Could you check a few things on this model? Use its own coordinates, in mm. A direction names the side the tool comes from. Coordinates: 2 decimals unless noted, no trailing zeros. Write each loop counter-clockwise with the first axis right and the second up, starting at its lowest first coordinate (ties: lowest second). Pieces come first, ordered by that corner, then holes.
Item 1: Which directions (+Z, -Z, +X, -X, +Y, -Y) give clear straight access to the entire face, cutting with the end or side of a thin tool? Please do faces 5 (the flat face through (4, 24, 34)), 6 (the flat face through (4, 29, -32)), 7 (the flat face through (4, 31.5, 0)).
Item 2: If I drill on probe 1 along Y at (x, z) = (4, 34.25); probe 2 along Z at (x, y) = (2, 30.5); probe 3 along Z at (x, y) = (5.75, 19.5), over which ranges is the centre line in solid material (lowest first)?
Item 3: I want a section at D-D on x = 4. State how many separate pieces and enclosed holes the cut face has, then the cut area to 3 significant figures.
Item 4: I want a section at C-C on y = 16. Please give me the cut outline in (x, z).
Item 5: I want a section at B-B on y = 30.75. Please give me the cut outline in (x, z), then the cut area to 3 significant figures.
Item 6: I want a section at A-A on z = -24. Please give me the cut outline in (x, y).
Item 7: Thinking about a two-plate mould opening in X: for faces 1 (the cylindrical face through (4, 10, 35)), 2 (the flat face through (8, 33, -2)), 3 (the flat face through (0, 33, -2)), 4 (the flat face through (4, 21, 31)), which applies, +X half, -X half, draft (parallel to the pull), parting line (faces both ways), or undercut?
Item 8: For P1, Ø2, axis at x = 6, z = -30.5, coming from the -Y side; P2, Ø3, axis at x = 3, y = 27.5, coming from the +Z side; P3, Ø8, axis at y = 17.5, z = -26.5, coming from the -X side; P4, Ø4, axis at x = 4, z = 24, coming from the -Y side, each with a flat end and sliding along its axis, tell me the tip position at first contact or that it passes through.
from build123d import *

# Parameters (mm, degrees)
F1_DEPTH = 8
F2_W     = 6.02
F2_H     = 5
F3_DEPTH = 72
F4_R     = 1.5
F5_DEPTH = 25
F6_R     = 2
F7_DEPTH = 72
F8_SIZE  = 1


with BuildPart() as f1:
    # F0 (on Right) → F1 (new body)
    with BuildSketch(Plane.YZ):
        Polygon((24, 36), (4, 36), (4, 33), (21, 33), (21, 29), (31.5, 29), (31.5, -29), (21, -29), (21, -33), (4, -33), (4, -36), (24, -36), (24, -32), (34, -32), (34, -15.6872682273), (34, 32), (24, 32), align=None)
    extrude(amount=F1_DEPTH)

    # F2 (on face) → F3 (cut)
    with BuildSketch(Plane.XY.offset(36)):
        with Locations((3.01, 1.5)):
            Rectangle(F2_W, F2_H)
    extrude(amount=-F3_DEPTH, mode=Mode.SUBTRACT)

    # F4 (on face) → F5 (cut)
    with BuildSketch(Plane(origin=(0, 34, 0), x_dir=(-1, 0, 0), z_dir=(0, 1, 0))):
        with Locations((-4, 24)):
            Circle(F4_R)
        with Locations((-4, -24)):
            Circle(F4_R)
    extrude(amount=-F5_DEPTH, mode=Mode.SUBTRACT)

    # F6 (on face) → F7 (cut)
    with BuildSketch(Plane.XY.offset(36)):
        with Locations((4, 16)):
            Circle(F6_R)
        with Locations((4, 8)):
            Circle(F6_R)
    extrude(amount=-F7_DEPTH, mode=Mode.SUBTRACT)

    # F8
    f8_edges = [f1.edges().sort_by_distance(p)[0] for p in [
        (8, 31.5, 0),
        (0, 31.5, 0),
        (8, 26.25, 29),
        (0, 26.25, 29),
        (8, 26.25, -29),
        (0, 26.25, -29),
    ]]
    chamfer(f8_edges, length=F8_SIZE)


solid = f1.part
Response values:
1. face 5: +Z, +X, -X, +Y
1. face 6: -Z, +X, -X, +Y
1. face 7: +X, -X, -Y
2. probe 1: y = 4 to 6, 10 to 14, 18 to 24
2. probe 2: z = -32 to -29, 29 to 32
2. probe 3: z = -36 to -33, 33 to 36
3. separate pieces: 7
3. enclosed holes: 0
3. area: 286 mm2
4. outline: (0, -36) - (2, -36) - (2, -33) - (0, -33) - close; (0, 33) - (2, 33) - (2, 36) - (0, 36) - close; (6, -36) - (8, -36) - (8, -33) - (6, -33) - close; (6, 33) - (8, 33) - (8, 36) - (6, 36) - close
5. outline: (0, -32) - (8, -32) - (8, -30) - (7, -29) - (1, -29) - (0, -30) - close; (0, 30) - (1, 29) - (7, 29) - (8, 30) - (8, 32) - (0, 32) - close
5. area: 46.0 mm2
6. outline: (0, 32.5) - (1, 31.5) - (2.5, 31.5) - (2.5, 34) - (0, 34) - close; (5.5, 31.5) - (7, 31.5) - (8, 32.5) - (8, 34) - (5.5, 34) - close
7. face 1: undercut
7. face 2: +X half
7. face 3: -X half
7. face 4: draft
8. P1: stops at y = 21
8. P2: stops at z = 32
8. P3: passes through
8. P4: stops at y = 31.5
